from build123d import *

# Parameters (mm, degrees)
F0_W     = 12.7
F0_H     = 50.8
F1_DEPTH = 101.6
F3_DEPTH = 12.701
F4_DEPTH = 165.1
F6_DEPTH = 177.801
F8_DEPTH = 177.801


with BuildPart() as f1:
    # F0 (on Front) → F1 (new body)
    with BuildSketch(Plane.XZ):
        Rectangle(F0_W, F0_H)
    extrude(amount=F1_DEPTH)

    # F2 (on face) → F3 (cut, through all)
    with BuildSketch(Plane.YZ.offset(6.35)):
        Polygon((-101.6, 25.4), (-101.6, -25.4), (-50.8, 25.4), align=None)
        Polygon((0, 25.4), (-50.8, 25.4), (0, -25.4), align=None)
    extrude(amount=-F3_DEPTH, mode=Mode.SUBTRACT)

    # F4 (add): a face of the model
    f4_faces = [f1.faces().sort_by_distance(p)[0] for p in [
        (-6.35, -50.8, -8.4666666667),
    ]]
    extrude(f4_faces, amount=F4_DEPTH)

    # F5 (on face) → F6 (cut, through all)
    with BuildSketch(Plane.YZ.offset(6.35)):
        Polygon((-50.7999999233, 12.7000000767), (-88.9, -25.4), (-12.6999998465, -25.4), align=None)
    extrude(amount=-F6_DEPTH, mode=Mode.SUBTRACT)

    # F7 (on face) → F8 (cut, through all)
    with BuildSketch(Plane.YZ.offset(6.35)):
        Polygon((-6.3499999233, -19.0500000767), (-12.6999998465, -25.4), (0, -25.4), align=None)
        Polygon((-101.6, -25.4), (-88.9, -25.4), (-95.25, -19.05), align=None)
    extrude(amount=-F8_DEPTH, mode=Mode.SUBTRACT)


solid = f1.part
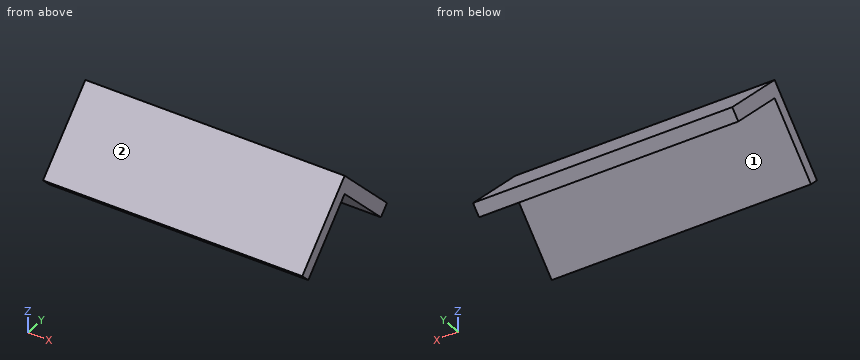
Verification items for the finished model (mm, model axes). Face numbers are marked on the shaded views. Round coordinates to 2 decimals unless told otherwise and drop trailing zeros. Loops run counter-clockwise (first coordinate to the right, second up) from the corner with the lowest first, then second, coordinate; pieces in that order, holes last. Notation, with made-up numbers: (33, 22.5) - (67, 22.5) arc R21 ccw to (67, 52.5) - close; hole circle Ø5 at (41, 73.5). An arc over 180 degrees is marked (long way). Use a Markdown table: item, result. Add a question column.
1. Section check D-D, the plane y = -64. Record the boundary of the cut face in (x, z).
2. Section check B-B, the plane x = -82.5. Record the boundary of the cut face in (y, z).
3. Gauge pin test, flat ends, axial feed: pin 1 (8 mm diameter, centred on x = -86.5, z = -4.5, fed in from +Y); pin 2 (8 mm diameter, centred on x = -19, y = -52.5, fed in from +Z); pin 3 (3 mm diameter, centred on x = -55, z = 2, fed in from -Y). Record the tip position at first contact, or that the pin passes through.
4. Release check for a two-part mould opening along Y. For the marked faces 1 and 2 record: released by +Y, released by -Y, zero draft, split by the parting line, or undercut.
5. Thickness scan on probe 1 along Y at (x, z) = (-3, 9); probe 2 along Y at (x, z) = (-128.5, -15.5); probe 3 along Z at (x, y) = (-17, -80.5). Record the ranges inside material, lowest first. Write a range as [from, to].
6. Section check C-C, the plane z = 8. Record the boundary of the cut face in (x, y).
7. Section check A-A, the plane z = -21. Record the boundary of the cut face in (x, y), plus the area to 3 significant figures.
Checks:
| question | item | result |
|---|---|---|
| 1 | outline | (-171.45, -0.5) - (6.35, -0.5) - (6.35, 12.2) - (-171.45, 12.2) - close |
| 2 | outline | (-95.25, -19.05) - (-88.9, -25.4) - (-50.8, 12.7) - (-12.7, -25.4) - (-6.35, -19.05) - (-50.8, 25.4) - close |
| 3 | pin 1 | stops at y = -16.9 |
| 3 | pin 2 | stops at z = 25.4 |
| 3 | pin 3 | stops at y = -75.7 |
| 4 | face 1 | undercut |
| 4 | face 2 | released by -Y |
| 5 | probe 1 | y = [-67.2, -54.5], [-47.1, -34.4] |
| 5 | probe 2 | y = [-91.7, -79], [-22.6, -9.9] |
| 5 | probe 3 | z = [-17, -4.3] |
| 6 | outline | (-171.45, -68.2) - (6.35, -68.2) - (6.35, -55.5) - (-171.45, -55.5) - close; (-171.45, -46.1) - (6.35, -46.1) - (6.35, -33.4) - (-171.45, -33.4) - close |
| 7 | outline | (-171.45, -93.3) - (6.35, -93.3) - (6.35, -84.5) - (-171.45, -84.5) - close; (-171.45, -17.1) - (6.35, -17.1) - (6.35, -8.3) - (-171.45, -8.3) - close |
| 7 | area | 3,130 mm^2 |
